Here's how the part is built. I have some questions about the finished solid (model axes, mm). Face numbers are marked on the shaded views. A direction names the side the tool comes from. Round coordinates to 2 decimals unless told otherwise and drop trailing zeros. Order: outer loops, then holes, each group sorted by start corner. A loop starts at its lowest first (then second) coordinate and runs counter-clockwise, first axis right, second up. Notation, with made-up numbers: (35.25, -32) -> (68.25, -32) arc R28 cw to (68.25, -4) -> close; hole circle Ø2 at (9.25, 7). An arc over 180 degrees is marked (long way). One line per item, written item: value.
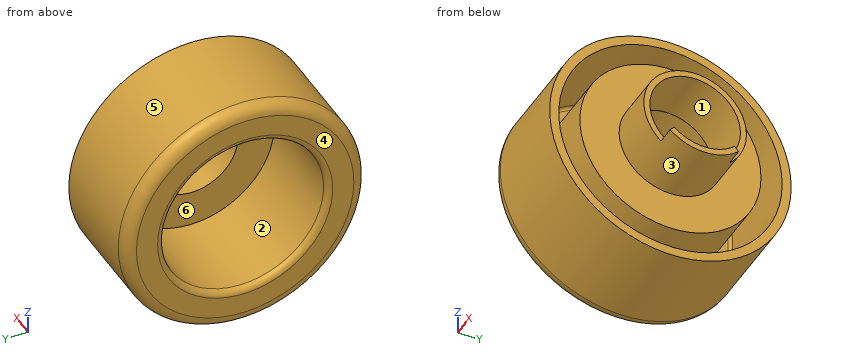
Autodesk Inventor part; units mm, degrees
ref_plane "Work Plane1" through (20, 0, 0) normal (1, 0, 0) x (0, 1, 0)
ref_plane "XZ Plane" through (0, 0, 0) normal (0, 1, 0) x (-1, 0, 0)
ref_plane "XY Plane" through (0, 0, 0) normal (0, 0, 1) x (1, 0, 0)
ref_plane "Work Plane1" through (20, 0, 0) normal (1, 0, 0) x (0, 1, 0)
sketch "Sketch7" plane through (0, 0, 0) normal (1, 0, 0) x (0, 1, 0)
  circle A0 centre (0, 0) radius 7.5
  circle A1 centre (0, 0) radius 20
  dimension "d28" = 15
  dimension "d29" = 40
extrude "Wheel" add sketch "Sketch7" along normal blind 18
sketch "Sketch8" plane through (0, 0, 0) normal (1, 0, 0) x (0, 1, 0)
  circle A0 centre (0, 0) radius 13.5
  dimension "d33" = 27
extrude "Extrusion7" cut sketch "Sketch8" along normal blind 17
fillet "Fillet1" radius 2 1 edges at (0, -20, 0)
fillet "Fillet2" radius 1 1 edges at (0, -13.5, 0)
shell "Shell1" thickness 1.5 removed faces 1 at (18, 15.6396, -1.5954)
sketch "Sketch10" plane through (18, 0, 0) normal (1, 0, 0) x (0, 0, -1)
  circle A0 centre (0, 0) radius 8.5
  circle A1 centre (0, 0) radius 7.5
  dimension "d41" = 17
extrude "Extrusion9" add sketch "Sketch10" along normal blind 8
sketch "Sketch12" plane through (26, 0, 0) normal (1, 0, 0) x (0, 0, -1)
  circle A0 centre (0, 0) radius 8.5
  circle A1 centre (0, 0) radius 7.5
  line L0 (0, 0) -> (5.5902, -5)
  line L1 (0, 0) -> (5.5902, 5)
  circle A2 centre (0, 0) radius 7.5
  line L2 (5.5902, 5) -> (5.5902, -5) construction
  line L3 (0, 0) -> (0, 5.0755) construction
  line L4 (5.5902, -5) -> (6.3355, -5.6667)
  line L5 (5.5902, 5) -> (6.3355, 5.6667)
  arc A3 (5.5902, -5) -> (5.5902, 5) centre (0, 0) ccw
  arc A4 (6.3355, -5.6667) -> (6.3355, 5.6667) centre (0, 0) ccw
  dimension "d53" = 10
extrude "Extrusion11" add sketch "Sketch12" along normal blind 3 contours A0 L4 A1 L5 picked at (8.0097, 1.2845)
properties part number "RearWheelRight"
Q1. I want a section at A-A on x = 15.5. Write out the boundary of the cut face in (y, z), then the cut area to 3 significant figures.
Answers:
outline: circle Ø40 at (0, 0); circle Ø30 at (0, 0); hole circle Ø37 at (0, 0); hole circle Ø27 at (0, 0)
area: 316 mm2
Q2. Which directions (+Z, -Z, +X, -X, +Y, -Y) give clear straight access to the entire face, cutting with the end or side of a thin tool? Please do the marked faces 1, 2 and 3.
Answers:
face 1: +X, -X
face 2: -X
face 3: +X
Q3. I want a section at B-B on x = 23. Write out the boundary of the cut face in (y, z).
Answers:
outline: circle Ø17 at (0, 0); hole circle Ø15 at (0, 0)
Q4. For P1, Ø12, axis at y = -7, z = -12, coming from the +X side; P2, Ø5, axis at x = 4, y = 9, coming from the +Z side; P3, Ø3, axis at x = 10, y = -7.5, coming from the +Z side; P4, Ø6, axis at y = -8.5, z = 9.5, coming from the +X side, each with a flat end and sliding along its axis, tell me the tip position at first contact or that it passes through.
Answers:
P1: x = 29
P2: z = 18.91
P3: z = 19.08
P4: x = 18
Q5. I need wall thicknesses on line 1 along Z through (x, y) = (9.75, 0); line 2 along Z through (x, y) = (21.25, 0); line 3 along Z through (x, y) = (17.5, 6.5). Which ranges of each line are inside material? Lowest first, please.
Answers:
line 1: -20 to -18.5, -15 to -13.5, 13.5 to 15, 18.5 to 20
line 2: -8.5 to -7.5, 7.5 to 8.5
line 3: -18.91 to -17.32, -13.52 to -3.74, 3.74 to 13.52, 17.32 to 18.91
Q6. If we mould it in two halves opening along Z, with no side actions, what happens to the marked faces 4, 5 and 6? For each: pulls with the +Z half, pulls with the -Z half, needs draft (parallel to the pull), parting line crosses it, or undercut.
Answers:
face 4: needs draft
face 5: parting line crosses it
face 6: undercut
